Input: part model. Units: mm. Frame: model coordinates. Face numbers are marked on the shaded views. A direction names the side the tool comes from. Give positions to 0.01 mm unless a question says otherwise; leave off trailing zeros. Loops run counter-clockwise (first coordinate to the right, second up) from the corner with the lowest first, then second, coordinate; pieces in that order, holes last. Notation, with made-up numbers: (23.25, 66.25) -> (81.25, 66.25) arc R31 cw to (81.25, 103.25) -> close; hole circle Ø3 at (-33.5, 37). An arc over 180 degrees is marked (long way). Answer as a JSON object with one key per item and string values.
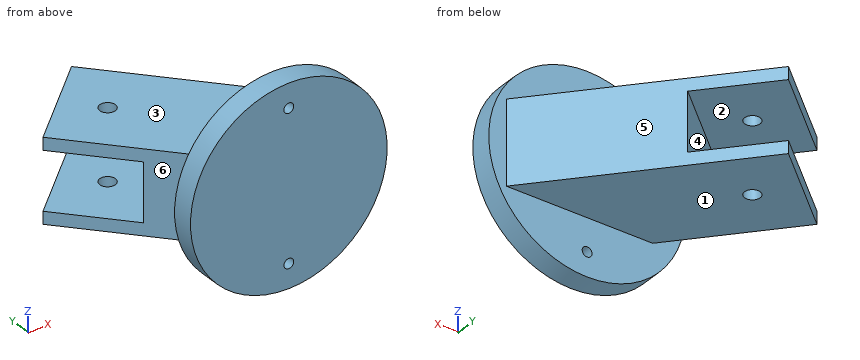
```python
from build123d import *

# Parameters (mm, degrees)
SKETCH1_R                = 45
SKETCH1_R_2              = 2.25
BOSS_EXTRUDE1_DEPTH      = 10
BOSS_EXTRUDE2_DEPTH      = 19.05
BOSS_EXTRUDE2_DEPTH_BACK = 19.05
SKETCH3_W                = 50
SKETCH3_H                = 26.67
CUT_EXTRUDE1_DEPTH       = 38.1
F_1_4_CLEARANCE_HOLE1_D  = 7.14248


with BuildPart() as part:
    # Sketch1 → Boss-Extrude1 (new body)
    with BuildSketch(Plane(origin=(0, 0, 0), x_dir=(1, 0, 0), z_dir=(0, 1, 0))):
        with Locations(Location((0, 0, 0), (0, 0, 270))):
            Circle(SKETCH1_R)
        with Locations(Location((0, 34, 0), (0, 0, 270))):
            Circle(SKETCH1_R_2, mode=Mode.SUBTRACT)
        with Locations(Location((0, -34, 0), (0, 0, 270))):
            Circle(SKETCH1_R_2, mode=Mode.SUBTRACT)
    extrude(amount=BOSS_EXTRUDE1_DEPTH)

    # Sketch2 → Boss-Extrude2 (add, two sides: drawn at the far end of the back side and taken through both)
    with BuildSketch(Plane.XY.offset(-BOSS_EXTRUDE2_DEPTH_BACK)):
        Polygon((36.966840414, 10), (-34.013367398, 89.666438803), (-71.345276512, 56.40492107), (-30, 10), align=None)
    extrude(amount=BOSS_EXTRUDE2_DEPTH + BOSS_EXTRUDE2_DEPTH_BACK)

    # Sketch3 → Cut-Extrude1 (cut)
    with BuildSketch(Plane(origin=(-59.588083083, 66.880198307, 0), x_dir=(0.7466381822853925, 0.6652303546543595, 0), z_dir=(-0.6652303546543595, 0.7466381822853925, 0))):
        with Locations((9.253158078, 0)):
            Rectangle(SKETCH3_W, SKETCH3_H)
    extrude(amount=-CUT_EXTRUDE1_DEPTH, mode=Mode.SUBTRACT)

    # 1_4 Clearance Hole1 (through all)
    with Locations(Plane.XY.offset(19.05)):
        with Locations((-40.006683699, 58.812222564)):
            Hole(F_1_4_CLEARANCE_HOLE1_D / 2)


solid = part.part
```
Q1. Section C-C, the plane y = 69.5. Return the cut outline in (x, z) (3 decimals), then the cut area to 3 significant figures.
Evaluation:
{"outline": "(-56.648, -19.05) -> (-16.046, -19.05) -> (-16.046, -13.335) -> (-56.648, -13.335) -> close; (-56.648, 13.335) -> (-16.046, 13.335) -> (-16.046, 19.05) -> (-56.648, 19.05) -> close", "area": "464 mm2"}
Q2. Access query for the marked faces 4, 5 and 6. Directions: +Z, -Z, +X, -X, +Y, -Y. A direction counts if a zero-diameter tool reaches every point of the face in a straight line with its end or side. Return the directions, or none.
Evaluation:
{"face 4": "-X, +Y", "face 5": "+Z, -Z, +X, +Y", "face 6": "+Z, -Z, -X"}
Q3. Ray query, line 1 along Z through (x, y) = (-60, 55) (3 decimals); line 2 along Z through (x, y) = (-12, 56); line 3 along X through (y, z) = (2, -34). Return the intervals inside material, ascending.
Evaluation:
{"line 1": "z = -19.05 to -13.335, 13.335 to 19.05", "line 2": "z = -19.05 to 19.05", "line 3": "x = -29.48 to -2.25, 2.25 to 29.48"}
Q4. Section B-B, the plane x = 0. Return the cut outline in (y, z), then the cut area to 3 significant figures.
Evaluation:
{"outline": "(0, -45) -> (10, -45) -> (10, -36.25) -> (0, -36.25) -> close; (0, -31.75) -> (10, -31.75) -> (10, -19.05) -> (51.49, -19.05) -> (51.49, 19.05) -> (10, 19.05) -> (10, 31.75) -> (0, 31.75) -> close; (0, 36.25) -> (10, 36.25) -> (10, 45) -> (0, 45) -> close", "area": "2,390 mm2"}
Q5. Section A-A, the plane z = 34. Return the cut outline in (x, y).
Evaluation:
{"outline": "(-29.48, 0) -> (-2.25, 0) -> (-2.25, 10) -> (-29.48, 10) -> close; (2.25, 0) -> (29.48, 0) -> (29.48, 10) -> (2.25, 10) -> close"}
Q6. Pin query (flat end, axial travel): pin 1 (4.5 mm diameter, centred on x = -40.01, y = 58.81, fed in from -Z); pin 2 (10 mm diameter, centred on x = -43, y = 74, fed in from -Z); pin 3 (12 mm diameter, centred on x = -34, y = 42.5, fed in from +Z); pin 4 (1 mm diameter, centred on y = 56, z = -6, fed in from +X). Return the tip coordinate at first contact, or that it passes through.
Evaluation:
{"pin 1": "passes through", "pin 2": "stops at z = -19.05", "pin 3": "stops at z = 19.05", "pin 4": "stops at x = -3.57"}
Q7. Draft query along Z for the marked faces 1, 2 and 3. Return one class per face: +Z half, -Z half, draft (parallel to the pull), parting line (faces both ways), or undercut.
Evaluation:
{"face 1": "-Z half", "face 2": "undercut", "face 3": "+Z half"}
